For this review, take the finished solid that the model builds, in its own axes (mm). A direction names the side the tool comes from. Round coordinates to 2 decimals unless told otherwise and drop trailing zeros. Loops run counter-clockwise (first coordinate to the right, second up) from the corner with the lowest first, then second, coordinate; pieces in that order, holes last.
```python
from build123d import *

# Parameters (mm, degrees)
BOX004_W               = 10
BOX004_H               = 12
BOX004_DEPTH           = 4
BOX003_W               = 35
BOX003_H               = 26.5
BOX003_DEPTH           = 10
BOX002_W               = 70
BOX002_H               = 19
BOX002_DEPTH           = 19
BOX002_PLACEMENT_ANGLE = 30
BOX001_W               = 70
BOX001_H               = 19
BOX001_DEPTH           = 19
BOX001_PLACEMENT_ANGLE = 90
BOX_W                  = 70
BOX_H                  = 19
BOX_DEPTH              = 19
BOX_PLACEMENT_ANGLE    = 30
PRISM001_DEPTH         = 19
PRISM_DEPTH            = 19


with BuildPart() as box004:
    # Box004 → Box004 (new body)
    with BuildSketch(Plane(origin=(84, -6, 15), x_dir=(1, 0, 0), z_dir=(0, 0, 1))):
        with Locations((5, 6)):
            Rectangle(BOX004_W, BOX004_H)
    extrude(amount=BOX004_DEPTH)


with BuildPart() as box003:
    # Box003 → Box003 (new body)
    with BuildSketch(Plane(origin=(93, -13.3, 9), x_dir=(1, 0, 0), z_dir=(0, 0, 1))):
        with Locations((17.5, 13.25)):
            Rectangle(BOX003_W, BOX003_H)
    extrude(amount=BOX003_DEPTH)


with BuildPart() as box002:
    # Box002 → Box002 (new body)
    with BuildSketch(Plane.XY):
        with Locations((35, 9.5)):
            Rectangle(BOX002_W, BOX002_H)
    extrude(amount=BOX002_DEPTH)


with BuildPart() as box002_1:
    # Box002 placement: moved
    add(box002.part.moved(Location((7, -82, 0))).rotate(Axis((7, -82, 0), (0, 0, 1)), BOX002_PLACEMENT_ANGLE))


with BuildPart() as box001:
    # Box001 → Box001 (new body)
    with BuildSketch(Plane.XY):
        with Locations((35, 9.5)):
            Rectangle(BOX001_W, BOX001_H)
    extrude(amount=BOX001_DEPTH)


with BuildPart() as box001_1:
    # Box001 placement: moved
    add(box001.part.moved(Location((-55, -35, 0))).rotate(Axis((-55, -35, 0), (0, 0, 1)), BOX001_PLACEMENT_ANGLE))


with BuildPart() as box:
    # Box → Box (new body)
    with BuildSketch(Plane.XY):
        with Locations((35, 9.5)):
            Rectangle(BOX_W, BOX_H)
    extrude(amount=BOX_DEPTH)


with BuildPart() as box_1:
    # Box placement: moved
    add(box.part.moved(Location((-2, 65, 0))).rotate(Axis((-2, 65, 0), (0, 0, -1)), BOX_PLACEMENT_ANGLE))


with BuildPart() as prism001:
    # Prism001 → Prism001 (new body)
    with BuildSketch(Plane.XY):
        Polygon((95, 0), (-47.5, 82.272413), (-47.5, -82.272413), align=None)
    extrude(amount=PRISM001_DEPTH)


with BuildPart() as cut005:
    # Prism → Prism (new body)
    with BuildSketch(Plane.XY):
        Polygon((165, 0), (-82.5, 142.894192), (-82.5, -142.894192), align=None)
    extrude(amount=PRISM_DEPTH)

    # Cut: cut Prism001
    add(prism001.part, mode=Mode.SUBTRACT)

    # Cut001: cut Box
    add(box_1.part, mode=Mode.SUBTRACT)

    # Cut002: cut Box001
    add(box001_1.part, mode=Mode.SUBTRACT)

    # Cut003: cut Box002
    add(box002_1.part, mode=Mode.SUBTRACT)

    # Cut004: cut Box003
    add(box003.part, mode=Mode.SUBTRACT)

    # Cut005: cut Box004
    add(box004.part, mode=Mode.SUBTRACT)


solid = cut005.part
```
(1) Add section A-A (z = 12). Give the boundary of the cut face in (x, y).
(2) Add section B-B (x = -65). Give the boundary of the cut face in (y, z).
(3) For faces 4 (the flat face through (93, 8, 13)), 5 (the flat face through (27.887, 47.745, 9.367)), 6 (the flat face through (42.98, 70.45, 9.37)), list the 3-axis set-ups (+Z, -Z, +X, -X, +Y, -Y) from which the entire face can be reached by the end or side of a thin tool; tool diameter is ignored.
(4) Insertion check: pin 1 Ø1 at (x, z) = (107, 8) entering from +Y (3 decimals); pin 2 Ø3 at (y, z) = (-10, 11.5) entering from +X; pin 3 Ø9.5 at (y, z) = (-20, 7) entering from +X; pin 4 Ø2 at (x, y) = (11, 77.5) entering from -Z. Each pin has a flat end and moves straight along its axis. Give the tip position at first contact, or say it passes through.
(5) The part is to be moulded in two halves that separate along X. For faces 1 (the flat face through (22, 43, 0)), 2 (the flat face through (39.518, -72.447, 9.367)), 3 (the flat face through (37.387, 64.199, 9.367)), say which applies: pulls with the +X half, pulls with the -X half, needs draft (parallel to the pull), parting line crosses it, or undercut.
(6) For L1, parallel to X at y = 17, z = 7.25; L2, parallel to Y at x = 32, z = 11.25; L3, parallel to X at y = -70, z = 9, list the stretches that pass through material, from the lowest coordinate up.
(7) Add section D-D (x = 14). Give the boundary of the cut face in (y, z), plus the area to 3 significant figures.
(8) Add section C-C (y = -21.5). Give the boundary of the cut face in (x, z), plus the area to 3 significant figures.
Outcome:
1. outline: (-82.5, -142.89) - (165, 0) - (-82.5, 142.89) - close; hole (-74, -35) - (-55, -35) - (-55, 35) - (-74, 35) - close; hole (-47.5, -82.27) - (93, -1.15) - (93, -13.3) - (128, -13.3) - (128, 13.2) - (93, 13.2) - (93, 1.15) - (-47.5, 82.27) - close; hole (-2.5, -65.55) - (7, -82) - (67.62, -47) - (58.12, -30.55) - close; hole (-2, 65) - (58.62, 30) - (68.12, 46.45) - (7.5, 81.45) - close
2. outline: (-132.79, 0) - (-35, 0) - (-35, 19) - (-132.79, 19) - close; (35, 0) - (132.79, 0) - (132.79, 19) - (35, 19) - close
3. face 4: +Z
3. face 5: +Z, -Z
3. face 6: +Z, -Z, +X, +Y
4. pin 1: stops at y = 33.775
4. pin 2: stops at x = 150.28
4. pin 3: stops at x = 138.59
4. pin 4: passes through
5. face 1: needs draft
5. face 2: pulls with the +X half
5. face 3: undercut
6. L1: x = -82.5 to -74, -55 to -47.5, 65.56 to 135.56
6. L2: y = -76.79 to -67.57, -45.63 to -36.37, 36.37 to 45.37, 67.31 to 76.79
6. L3: x = -82.5 to -47.5, -26.24 to 0.07, 27.78 to 43.76
7. outline: (-87.18, 0) - (-77.96, 0) - (-77.96, 19) - (-87.18, 19) - close; (-56.02, 0) - (-46.77, 0) - (-46.77, 19) - (-56.02, 19) - close; (46.77, 0) - (55.76, 0) - (55.76, 19) - (46.77, 19) - close; (77.7, 0) - (87.18, 0) - (87.18, 19) - (77.7, 19) - close
7. area: 702 mm2
8. outline: (-82.5, 0) - (-74, 0) - (-74, 19) - (-82.5, 19) - close; (-55, 0) - (-47.5, 0) - (-47.5, 19) - (-55, 19) - close; (57.76, 0) - (127.76, 0) - (127.76, 19) - (57.76, 19) - close
8. area: 1,630 mm2
